Source: three-view drawing plus pictorial views. Frame: mm from the lowest corner of the part. A direction names the side the tool comes from. Coordinates: 2 decimals unless noted, no trailing zeros. Loops run counter-clockwise (first coordinate to the right, second up) from the corner with the lowest first, then second, coordinate; pieces in that order, holes last. Notation, with made-up numbers: (19, 56.5) - (50, 56.5) arc R15 cw to (50, 61.5) - close; hole circle Ø1 at (-37, 6). An arc over 180 degrees is marked (long way). Return JSON: item names as keys, results as strings.
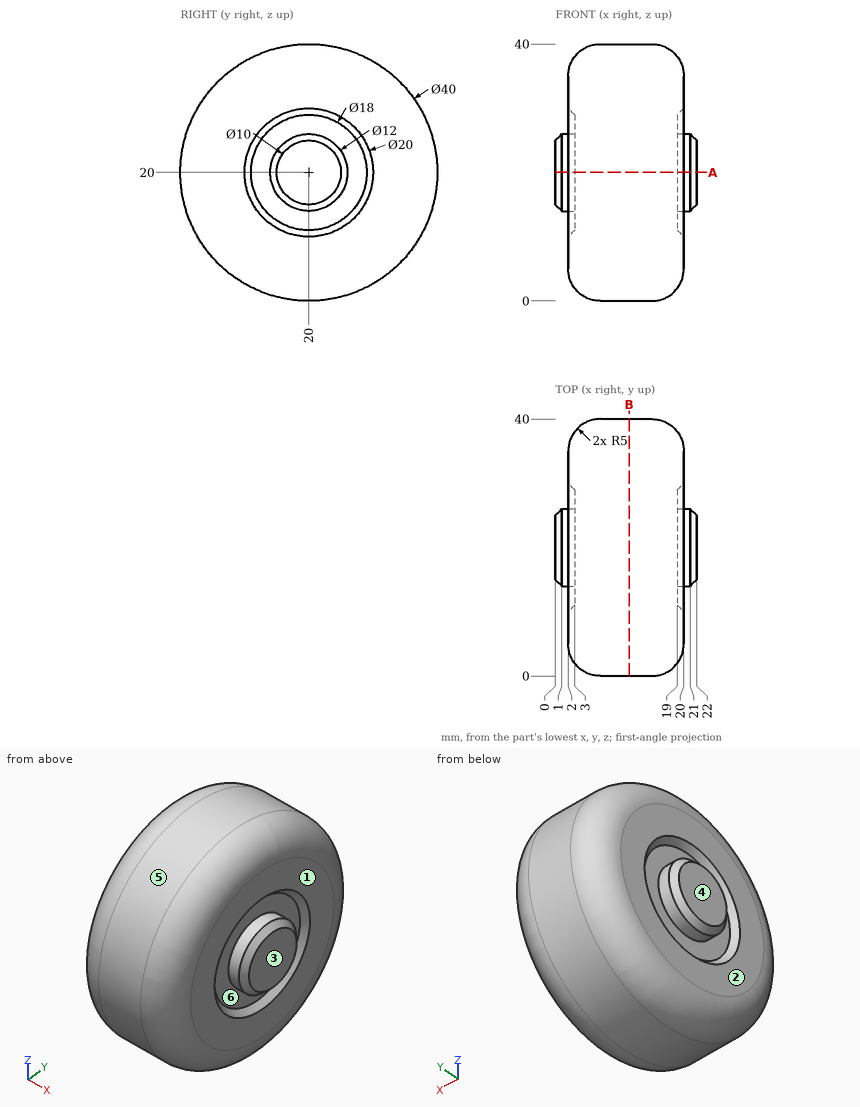
Item 1: Section query A-A, the plane z = 20. Return loops of the section in (x, y), and give its area (3 significant figures).
Worked out:
{"outline": "(0, 15) - (1, 14) - (3, 14) - (3, 11) - (2, 10) - (2, 5) arc R5 ccw to (7, 0) - (15, 0) arc R5 ccw to (20, 5) - (20, 10) - (19, 11) - (19, 14) - (21, 14) - (22, 15) - (22, 25) - (21, 26) - (19, 26) - (19, 29) - (20, 30) - (20, 35) arc R5 ccw to (15, 40) - (7, 40) arc R5 ccw to (2, 35) - (2, 30) - (3, 29) - (3, 26) - (1, 26) - (0, 25) - close", "area": "731 mm^2"}
Item 2: Reachability of the marked faces 1, 2 and 3 from +Z, -Z, +X, -X, +Y, -Y: full face, straight path, thin tool, end or side. Return the list, or none.
Worked out:
{"face 1": "+X", "face 2": "-X", "face 3": "+Z, -Z, +X, +Y, -Y"}
Item 3: Mould query, pull axis Z, two halves, no side actions, for the marked faces 4, 5 and 6. Classes: +Z half, -Z half, draft (parallel to the pull), parting line (faces both ways), or undercut.
Worked out:
{"face 4": "draft", "face 5": "parting line", "face 6": "undercut"}
Item 4: First-contact query: pin 1 Ø1 at (y, z) = (20, 29) entering from -X; pin 2 Ø1 at (y, z) = (21.5, 10.5) entering from -X; pin 3 Ø1.5 at (x, z) = (6.5, 7.5) entering from +Y. Flat tips, straight axial feed; report the tip coordinate or a pass-through.
Worked out:
{"pin 1": "x = 2.5", "pin 2": "x = 2", "pin 3": "y = 36.16"}
Item 5: Ray query, probe 1 along Z at (x, y) = (19.5, 19.5); probe 2 along X at (y, z) = (32, 21); probe 3 along Y at (x, z) = (2.5, 28). Return the intervals inside material, ascending. Write a range as from..to.
Worked out:
{"probe 1": "2.83..10.51, 14.02..25.98, 29.49..37.17", "probe 2": "2..20", "probe 3": "4.8..14.88, 25.12..35.2"}
Item 6: Section query B-B, the plane x = 11.5. Return loops of the section in (y, z).
Worked out:
{"outline": "circle Ø40 at (20, 20)"}
